Could you check a few things on this model? Use its own coordinates, in mm. Face numbers are marked on the shaded views. A direction names the side the tool comes from. Coordinates: 2 decimals unless noted, no trailing zeros. Loops run counter-clockwise (first coordinate to the right, second up) from the corner with the lowest first, then second, coordinate; pieces in that order, holes last. Notation, with made-up numbers: M 17.5,72 L 57.5,72 A33 cw 57.5,108 Z; hole C -5.75,10 d10. An arc over 180 degrees is marked long. Return JSON: item names as keys, results as strings. Group by question number.
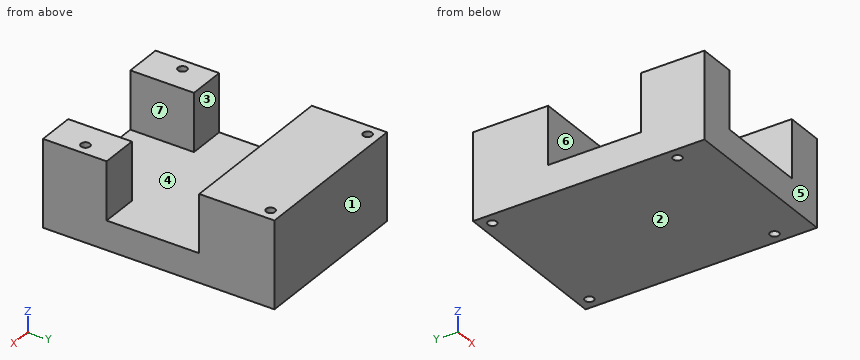
from build123d import *

# Parameters (mm, degrees)
F0_W     = 29
F0_H     = 40
F0_R     = 0.765
F1_DEPTH = 15
F2_W     = 29
F2_H     = 16
F3_DEPTH = 10
F4_W     = 16
F4_H     = 10
F5_DEPTH = 25


with BuildPart() as f1:
    # F0 (on Top) → F1 (new body)
    with BuildSketch(Plane.XY):
        Rectangle(F0_W, F0_H)
        with Locations((-12.5, -14)):
            Circle(F0_R, mode=Mode.SUBTRACT)
        with Locations((12.5, -14)):
            Circle(F0_R, mode=Mode.SUBTRACT)
        with Locations((-12.5, 18)):
            Circle(F0_R, mode=Mode.SUBTRACT)
        with Locations((12.5, 18)):
            Circle(F0_R, mode=Mode.SUBTRACT)
    extrude(amount=F1_DEPTH)

    # F2 (on face) → F3 (cut)
    with BuildSketch(Plane.XY.offset(15)):
        with Locations((0, -1)):
            Rectangle(F2_W, F2_H)
    extrude(amount=-F3_DEPTH, mode=Mode.SUBTRACT)

    # F4 (on face) → F5 (cut)
    with BuildSketch(Plane.XZ.offset(20)):
        with Locations((0, 10)):
            Rectangle(F4_W, F4_H)
    extrude(amount=-F5_DEPTH, mode=Mode.SUBTRACT)


solid = f1.part
(1) For the marked faces 5, 6 and 7, which set-ups out of +Z, -Z, +X, -X, +Y, -Y let a thin tool reach every point of the face, with its end or its side?
(2) Imagine slicing it at C-C, the plane y = 18. Write out the boundary of the cut face in (x, z) (3 decimals).
(3) Will these pins go through, and if not, where does the flat tip stop? P1, Ø1.2, axis at x = 12.5, y = 18, coming from the +Z side; P2, Ø8, axis at x = 6.5, y = -4, coming from the +Z side.
(4) Imagine slicing it at A-A, the plane z = 6.5. Write out the boundary of the cut face in (x, y) (3 decimals).
(5) Imagine slicing it at D-D, the plane y = -14. Write out the boundary of the cut face in (x, z) (3 decimals).
(6) If I drill on L1, parallel to Y at x = -12.5, z = 11.25 (3 decimals); L2, parallel to Y at x = 12.5, z = 4.75 (3 decimals); L3, parallel to Y at x = 8.75, z = 14.25, over which ranges is the centre line in solid material (lowest first)? Write a range as [from, to].
(7) Imagine slicing it at B-B, the plane x = 12.5. Write out the boundary of the cut face in (y, z) (3 decimals), then the cut area to 3 significant figures.
(8) We'd pull the mould along Y, two halves only. Please class the marked faces 1, 2, 3 and 4: +Y half, -Y half, draft (parallel to the pull), parting line (faces both ways), or undercut.
Checks:
{
 "1": {"face 5": "+Z, -Z, +X, -X, -Y", "face 6": "+Z, +X, -X", "face 7": "+Z, -Y"},
 "2": {"outline": "M -14.5,0 L -13.265,0 L -13.265,15 L -14.5,15 Z; M -11.735,0 L 11.735,0 L 11.735,15 L -11.735,15 Z; M 13.265,0 L 14.5,0 L 14.5,15 L 13.265,15 Z"},
 "3": {"P1": "through", "P2": "z = 5"},
 "4": {"outline": "M -14.5,-20 L -8,-20 L -8,-9 L -14.5,-9 Z; M -14.5,7 L 14.5,7 L 14.5,20 L -14.5,20 Z; M 8,-20 L 14.5,-20 L 14.5,-9 L 8,-9 Z; hole C -12.5,-14 d1.53; hole C -12.5,18 d1.53; hole C 12.5,-14 d1.53; hole C 12.5,18 d1.53"},
 "5": {"outline": "M -14.5,0 L -13.265,0 L -13.265,15 L -14.5,15 Z; M -11.735,0 L 11.735,0 L 11.735,15 L 8,15 L 8,5 L -8,5 L -8,15 L -11.735,15 Z; M 13.265,0 L 14.5,0 L 14.5,15 L 13.265,15 Z"},
 "6": {"L1": "[-20, -14.765], [-13.235, -9], [7, 17.235], [18.765, 20]", "L2": "[-20, -14.765], [-13.235, 17.235], [18.765, 20]", "L3": "[-20, -9], [7, 20]"},
 "7": {"outline": "M -20,0 L -14.765,0 L -14.765,15 L -20,15 Z; M -13.235,0 L 17.235,0 L 17.235,15 L 7,15 L 7,5 L -9,5 L -9,15 L -13.235,15 Z; M 18.765,0 L 20,0 L 20,15 L 18.765,15 Z", "area": "394 mm²"},
 "8": {"face 1": "+Y half", "face 2": "draft", "face 3": "undercut", "face 4": "undercut"}
}
